from build123d import *

# Parameters (mm, degrees)
SKETCH1_W                 = 50.8
SKETCH1_H                 = 25.4
SKETCH1_W_2               = 44.45
SKETCH1_H_2               = 19.05
BOSS_EXTRUDE1_DEPTH       = 227.0125
SKETCH2_W                 = 25.4
SKETCH2_H                 = 25.4
CUT_EXTRUDE1_DEPTH        = 230.836888154
F_8_32_TAPPED_HOLE1_D     = 3.4544
CUT_EXTRUDE2_DEPTH        = 230.836888154
FILLET1_R                 = 3.175
F_8_32_TAPPED_HOLE2_D     = 3.4544
F_8_32_TAPPED_HOLE2_DEPTH = 3.175
F_8_32_TAPPED_HOLE3_D     = 3.4544


with BuildPart() as part:
    # Sketch1 → Boss-Extrude1 (new, symmetric)
    with BuildSketch(Plane(origin=(0, 0, 0), x_dir=(0, 0, -1), z_dir=(1, 0, 0))):
        Rectangle(SKETCH1_W, SKETCH1_H)
        Rectangle(SKETCH1_W_2, SKETCH1_H_2, mode=Mode.SUBTRACT)
    extrude(amount=BOSS_EXTRUDE1_DEPTH, both=True)

    # Sketch2 → Cut-Extrude1 (cut, through all)
    with BuildSketch(Plane.XZ.offset(12.7)):
        with Locations((-214.3125, -12.7)):
            Rectangle(SKETCH2_W, SKETCH2_H)
    extrude(amount=-CUT_EXTRUDE1_DEPTH, mode=Mode.SUBTRACT)

    # #8-32 Tapped Hole1 (through all)
    with Locations(Plane(origin=(0, -12.7, 0), x_dir=(-1, 0, 0), z_dir=(0, -1, 0))):
        with Locations((-214.3125, 19.05), (-214.3125, -19.05), (-201.6125, 0), (188.9125, 12.7), (188.9125, -12.7), (214.3125, -12.7)):
            Hole(F_8_32_TAPPED_HOLE1_D / 2)

    # Sketch7 → Cut-Extrude2 (cut, through all)
    with BuildSketch(Plane(origin=(0, 12.7, 0), x_dir=(1, 0, 0), z_dir=(0, 1, 0))):
        Polygon((-176.2125, 15.875), (-130.571875, 15.875), (-176.2125, -15.875), align=None)
        Polygon((-148.828125, -15.875), (-103.1875, 15.875), (-57.546875, -15.875), align=None)
        Polygon((-75.803125, 15.875), (-30.1625, -15.875), (15.478125, 15.875), align=None)
        Polygon((42.8625, 15.875), (88.503125, -15.875), (-2.778125, -15.875), align=None)
        Polygon((70.246875, 15.875), (161.528125, 15.875), (115.8875, -15.875), align=None)
        Polygon((143.271875, -15.875), (188.9125, 15.875), (188.9125, -15.875), align=None)
    extrude(amount=-CUT_EXTRUDE2_DEPTH, mode=Mode.SUBTRACT)

    # Fillet1
    fillet1_edges = [part.edges().sort_by_distance(p)[0] for p in [
        (-176.2125, 11.1125, 15.875),
        (-176.2125, 11.1125, -15.875),
        (-130.571875, 11.1125, -15.875),
        (-176.2125, -11.1125, 15.875),
        (-176.2125, -11.1125, -15.875),
        (-130.571875, -11.1125, -15.875),
        (-57.546875, 11.1125, 15.875),
        (-148.828125, 11.1125, 15.875),
        (-103.1875, 11.1125, -15.875),
        (-57.546875, -11.1125, 15.875),
        (-148.828125, -11.1125, 15.875),
        (-103.1875, -11.1125, -15.875),
        (-75.803125, 11.1125, -15.875),
        (15.478125, 11.1125, -15.875),
        (-30.1625, 11.1125, 15.875),
        (-75.803125, -11.1125, -15.875),
        (15.478125, -11.1125, -15.875),
        (-30.1625, -11.1125, 15.875),
        (-2.778125, 11.1125, 15.875),
        (42.8625, 11.1125, -15.875),
        (88.503125, 11.1125, 15.875),
        (-2.778125, -11.1125, 15.875),
        (42.8625, -11.1125, -15.875),
        (88.503125, -11.1125, 15.875),
        (115.8875, 11.1125, 15.875),
        (70.246875, 11.1125, -15.875),
        (161.528125, 11.1125, -15.875),
        (115.8875, -11.1125, 15.875),
        (70.246875, -11.1125, -15.875),
        (161.528125, -11.1125, -15.875),
        (188.9125, 11.1125, 15.875),
        (143.271875, 11.1125, 15.875),
        (188.9125, 11.1125, -15.875),
        (188.9125, -11.1125, 15.875),
        (143.271875, -11.1125, 15.875),
        (188.9125, -11.1125, -15.875),
    ]]
    fillet(fillet1_edges, radius=FILLET1_R)

    # #8-32 Tapped Hole2
    with Locations(Plane(origin=(0, 0, -25.4), x_dir=(-1, 0, 0), z_dir=(0, 0, -1))):
        with Locations((176.2125, 0), (125.4125, 0), (74.6125, 0), (23.8125, 0), (-26.9875, 0), (-77.7875, 0), (-128.5875, 0), (-179.3875, 0)):
            Hole(F_8_32_TAPPED_HOLE2_D / 2, depth=F_8_32_TAPPED_HOLE2_DEPTH)

    # #8-32 Tapped Hole3 (through all)
    with Locations(Plane(origin=(0, 12.7, 0), x_dir=(1, 0, 0), z_dir=(0, 1, 0))):
        with Locations((185.7375, 19.05), (185.7375, -19.05)):
            Hole(F_8_32_TAPPED_HOLE3_D / 2)


solid = part.part
The model under review builds one solid part; all positions refer to its coordinate system, in mm. A direction names the side the tool comes from. Round coordinates to 2 decimals unless told otherwise and drop trailing zeros. Use one line per item in the form item = value.
Q1. Tool access review of faces 1 (the flat face through (3, 0, 22.225)), 2 (the flat face through (16, 0, -25.4)), 3 (the flat face through (62.19, 11.13, -2.43)): name each direction out of +Z, -Z, +X, -X, +Y, -Y from which nothing blocks a thin tool from reaching the whole face with its end or side.
Response values:
face_1 = +X, -X
face_2 = -Z, +X, -X, +Y, -Y
face_3 = +Y, -Y
Q2. Clearance check with flat-ended pins moving along their axes: P1, Ø6, axis at y = -9.5, z = -1.5, coming from the +X side; P2, Ø1, axis at x = -214.5, y = 10.5, coming from the -Z side. State where each tip first meets the part, or that it passes through.
Response values:
P1 = 227.01
P2 = 0
Q3. To check wall thickness, follow line 1 (X direction, y = -10.9, z = -19.05); line 2 (Z direction, x = -95, y = -10.25) (3 decimals); line 3 (Z direction, x = -67.5, y = 3.75) (3 decimals). State the ranges of each line that lie inside material, in increasing order.
Response values:
line_1 = -201.61 to 184.01, 187.46 to 212.59, 216.04 to 227.01
line_2 = -25.4 to -10.179, 15.875 to 25.4
line_3 = -25.4 to -22.225, 22.225 to 25.4
Q4. Mouldability with a two-part tool opening along Y and no side actions: class faces 4 (the flat face through (3, 12.7, 0)), 5 (the flat face through (62.19, -11.09, -2.43)), 6 (the flat face through (16, 0, -22.225)) as pulls with the +Y half, pulls with the -Y half, needs draft (parallel to the pull), parting line crosses it, or undercut.
Response values:
face_4 = pulls with the +Y half
face_5 = needs draft
face_6 = undercut
